```python
from build123d import *

# Parameters (mm, degrees)
SKETCH013_R         = 0.5
PAD006_DEPTH        = 2.6
SKETCH014_R         = 3
SKETCH014_R_2       = 0.5
PAD007_DEPTH        = 4
HOLE007_D           = 2.3
HOLE007_CSINK_D     = 3.3
HOLE007_CSINK_ANGLE = 90
HOLE008_D           = 3.2
HOLE008_CBORE_D     = 6
HOLE008_CBORE_DEPTH = 1.7
POCKET_DEPTH        = 132.355359


with BuildPart() as part:
    # Sketch013 → Pad006 (new body)
    with BuildSketch(Plane.XY):
        with BuildLine():
            ThreePointArc((-27, 11.89), (-29.12132, 11.01132), (-30, 8.89))
            Line((-30, -8.89), (-30, 8.89))
            ThreePointArc((-30, -8.89), (-29.12132, -11.01132), (-27, -11.89))
            Line((27, -11.89), (-27, -11.89))
            ThreePointArc((27, -11.89), (29.12132, -11.01132), (30, -8.89))
            Line((30, 8.89), (30, -8.89))
            ThreePointArc((30, 8.89), (29.12132, 11.01132), (27, 11.89))
            Line((-27, 11.89), (27, 11.89))
        make_face()
        with Locations((-22.86, 8.89)):
            Circle(SKETCH013_R, mode=Mode.SUBTRACT)
        with Locations((22.86, 8.89)):
            Circle(SKETCH013_R, mode=Mode.SUBTRACT)
        with Locations((22.86, -8.89)):
            Circle(SKETCH013_R, mode=Mode.SUBTRACT)
        with Locations((-22.86, -8.89)):
            Circle(SKETCH013_R, mode=Mode.SUBTRACT)
    extrude(amount=PAD006_DEPTH)

    # Sketch014 (on Face14 of Pad006) → Pad007 (join)
    with BuildSketch(Plane.XY.offset(2.6)):
        with Locations((-22.86, 8.89)):
            Circle(SKETCH014_R)
        with Locations((-22.86, 8.89)):
            Circle(SKETCH014_R_2, mode=Mode.SUBTRACT)
        with Locations((22.86, 8.89)):
            Circle(SKETCH014_R)
        with Locations((22.86, 8.89)):
            Circle(SKETCH014_R_2, mode=Mode.SUBTRACT)
        with Locations((-22.86, -8.89)):
            Circle(SKETCH014_R)
        with Locations((-22.86, -8.89)):
            Circle(SKETCH014_R_2, mode=Mode.SUBTRACT)
        with Locations((22.86, -8.89)):
            Circle(SKETCH014_R)
        with Locations((22.86, -8.89)):
            Circle(SKETCH014_R_2, mode=Mode.SUBTRACT)
    extrude(amount=PAD007_DEPTH)

    # Hole007 (through all)
    with Locations(Plane.XY.offset(6.6)):
        with Locations((-22.86, 8.89), (22.86, 8.89), (22.86, -8.89), (-22.86, -8.89)):
            CounterSinkHole(HOLE007_D / 2, HOLE007_CSINK_D / 2, counter_sink_angle=HOLE007_CSINK_ANGLE)

    # Hole008 (through all)
    with Locations(Plane.XY.offset(2.6)):
        with Locations((-25.5, 0), (25.5, 0)):
            CounterBoreHole(HOLE008_D / 2, HOLE008_CBORE_D / 2, HOLE008_CBORE_DEPTH)

    # Sketch017 (on Face5 of Hole008) → Pocket (cut, through all)
    with BuildSketch(Plane.XY.offset(2.6)):
        with BuildLine():
            ThreePointArc((-22.86, 11.89), (-24.98132, 11.01132), (-25.86, 8.89))
            ThreePointArc((-28.396031, 3.444271), (-26.525094, 5.88636), (-25.86, 8.89))
            ThreePointArc((-28.396031, 3.444271), (-30, 0), (-28.396031, -3.444271))
            ThreePointArc((-25.86, -8.89), (-26.525094, -5.88636), (-28.396031, -3.444271))
            ThreePointArc((-25.86, -8.89), (-24.98132, -11.01132), (-22.86, -11.89))
            Line((-32.97494, -11.89), (-22.86, -11.89))
            Line((-32.97494, -8.89), (-32.97494, -11.89))
            Line((-32.97494, 8.89), (-32.97494, -8.89))
            Line((-32.97494, 8.89), (-32.97494, 11.89))
            Line((-32.97494, 11.89), (-22.86, 11.89))
        make_face()
    pocket = extrude(amount=-POCKET_DEPTH, mode=Mode.SUBTRACT)

    # Mirrored005: Pocket across Sketch017 V_Axis
    add(pocket.mirror(Plane(origin=(0, 0, 2.6), x_dir=(0, 0, 1), z_dir=(1, 0, 0))), mode=Mode.SUBTRACT)


solid = part.part
```
The model under review builds one solid part; all positions refer to its coordinate system, in mm. A direction names the side the tool comes from. Give positions to 0.01 mm unless a question says otherwise; leave off trailing zeros. Write each loop counter-clockwise with the first axis right and the second up, starting at its lowest first coordinate (ties: lowest second). Pieces come first, ordered by that corner, then holes. Notation, with made-up numbers: (-5.75, 9) - (40.25, 9) arc R20 ccw to (40.25, 30) - close; hole circle Ø7 at (41.5, -3). An arc over 180 degrees is marked (long way). Answer in a Markdown table with one row per item. Add a question column.
1. We need section A-A on z = 4.5. Write out the cut boundary in (x, y).
2. We need section B-B on y = 0. Write out the cut boundary in (x, z), then the cut area to 3 significant figures.
3. We need section C-C on z = 2. Write out the cut boundary in (x, y), then the cut area to 3 significant figures.
4. Draft analysis for pull direction Y (two halves, no side actions). For faces 3 (the cylindrical face through (-30, 0, 1)), 4 (the cylindrical face through (-23.922, -9.33, 3.007)), 5 (the cylindrical face through (26.54, 5.85, 1.32)), state which applies: +Y half, -Y half, draft (parallel to the pull), parting line (faces both ways), or undercut.
5. Wall thickness on line 1 along X through (y, z) = (-8.89, 3.75); line 2 along X through (y, z) = (-9, 2); line 3 along Y through (x, z) = (22.86, 3): over which ranges is each line inside the solid? List them lowest first. Write a range as [from, to].
6. Tool access review of faces 1 (the cylindrical face through (-28.5, 0.1, 1.8)), 2 (the cylindrical face through (-26.507, -5.926, 1.318)): name each direction out of +Z, -Z, +X, -X, +Y, -Y from which nothing blocks a thin tool from reaching the whole face with its end or side.
7. Insertion check: P1, Ø2.5, axis at x = -22.86, y = -8.89, coming from the +Z side; P2, Ø1, axis at x = 5.5, y = 0, coming from the +Z side; P3, Ø5, axis at x = -25.5, y = 0, coming from the +Z side. Each pin has a flat end and moves straight along its axis. Give the tip position at first contact, or say it passes through.
8. We need section D-D on x = -15.5. Write out the cut boundary in (y, z).
Ans:
| question | item | result |
|---|---|---|
| 1 | outline | circle Ø6 at (-22.86, -8.89); circle Ø6 at (-22.86, 8.89); circle Ø6 at (22.86, -8.89); circle Ø6 at (22.86, 8.89); hole circle Ø2.3 at (-22.86, -8.89); hole circle Ø2.3 at (-22.86, 8.89); hole circle Ø2.3 at (22.86, -8.89); hole circle Ø2.3 at (22.86, 8.89) |
| 2 | outline | (-30, 0) - (-27.1, 0) - (-27.1, 0.9) - (-28.5, 0.9) - (-28.5, 2.6) - (-30, 2.6) - close; (-23.9, 0) - (23.9, 0) - (23.9, 0.9) - (22.5, 0.9) - (22.5, 2.6) - (-22.5, 2.6) - (-22.5, 0.9) - (-23.9, 0.9) - close; (27.1, 0) - (30, 0) - (30, 2.6) - (28.5, 2.6) - (28.5, 0.9) - (27.1, 0.9) - close |
| 2 | area | 130 mm^2 |
| 3 | outline | (-28.4, -3.44) arc R7.11 cw to (-25.86, -8.89) arc R3 ccw to (-22.86, -11.89) - (22.86, -11.89) arc R3 ccw to (25.86, -8.89) arc R7.11 cw to (28.4, -3.44) arc R4.5 ccw to (28.4, 3.44) arc R7.11 cw to (25.86, 8.89) arc R3 ccw to (22.86, 11.89) - (-22.86, 11.89) arc R3 ccw to (-25.86, 8.89) arc R7.11 cw to (-28.4, 3.44) arc R4.5 ccw to start; hole circle Ø6 at (-25.5, 0); hole circle Ø2.3 at (-22.86, -8.89); hole circle Ø2.3 at (-22.86, 8.89); hole circle Ø2.3 at (22.86, -8.89); hole circle Ø2.3 at (22.86, 8.89); hole circle Ø6 at (25.5, 0) |
| 3 | area | 1,220 mm^2 |
| 4 | face 3 | parting line |
| 4 | face 4 | undercut |
| 4 | face 5 | +Y half |
| 5 | line 1 | x = [-25.86, -24.01], [-21.71, -19.86], [19.86, 21.71], [24.01, 25.86] |
| 5 | line 2 | x = [-25.86, -24], [-21.72, 21.72], [24, 25.86] |
| 5 | line 3 | y = [-11.89, -10.04], [-7.74, -5.89], [5.89, 7.74], [10.04, 11.89] |
| 6 | face 1 | +Z |
| 6 | face 2 | +Z, -Z, -X, -Y |
| 7 | P1 | stops at z = 6.2 |
| 7 | P2 | stops at z = 2.6 |
| 7 | P3 | stops at z = 0.9 |
| 8 | outline | (-11.89, 0) - (11.89, 0) - (11.89, 2.6) - (-11.89, 2.6) - close |
